CAD build for the part. Positions are in the model's coordinates, mm. A direction names the side the tool comes from. Round coordinates to 2 decimals unless told otherwise and drop trailing zeros. Write each loop counter-clockwise with the first axis right and the second up, starting at its lowest first coordinate (ties: lowest second). Pieces come first, ordered by that corner, then holes. Notation, with made-up numbers: (8, -34) - (14, -34) arc R7 ccw to (14, -22) - close; hole circle Ø9 at (13.5, -18.5). An arc over 180 degrees is marked (long way). Use one line per item in the form item = value. Start each with the question number.
Item 1: Drill centre lines: L1, parallel to Z at x = 15, y = 5.75; L2, parallel to Y at x = 27.5, z = -14.5. Where is each one in solid material? Low to high.
Item 2: Tool access for faces 4 (the cylindrical face through (9.4, 99.43, -24.65)), 5 (the cylindrical face through (15.18, 39.4, -34.43)), 6 (the cylindrical face through (12.05, 6.59, -20.2)), 7 (the cylindrical face through (0.57, 50.56, -10.29)): list every direction of +Z, -Z, +X, -X, +Y, -Y with a clear straight run to the whole face (end or side of a thin tool).
Item 3: Pull direction X, two halves, no side cores. Call faces 1 (the flat face through (15, 48, -50)), 2 (the cylindrical face through (0.6, 14.43, -17.28)), 3 (the flat face through (20, 86, -25)): +X half, -X half, draft (parallel to the pull), parting line (faces both ways), or undercut.
Item 4: Band-saw the part on B-B, the plane x = 4. List the corners of the cut face in (y, z).
Item 5: Pin check, flat tips, straight feed: pin 1 (13.5 mm diameter, centred on x = 17, z = -27.5, fed in from -Y); pin 2 (10.5 mm diameter, centred on x = 11.5, y = 30.5, fed in from +Z); pin 3 (6.5 mm diameter, centred on x = 15, z = -17.5, fed in from +Y). Stop position of each tip, or through.
Item 6: Band-saw the part on D-D, the plane z = -15. Give the number of separate pieces and of enclosed holes in the cut face, and give its area (3 significant figures).
Item 7: Band-saw the part on A-A, the plane y = 90. List the corners of the cut face in (x, z).
Item 8: Band-saw the part on C-C, the plane x = 15. List the corners of the cut face in (y, z), and give its area (3 significant figures).
from build123d import *

# Parameters (mm, degrees)
BOSS_EXTRUDE1_DEPTH = 30
SKETCH3_R           = 4
CUT_EXTRUDE1_DEPTH  = 30
SKETCH4_W           = 10
SKETCH4_H           = 50
CUT_EXTRUDE2_DEPTH  = 51
SKETCH5_R           = 2.5
CUT_EXTRUDE3_DEPTH  = 30
FILLET1_R           = 2
CUT_EXTRUDE4_DEPTH  = 31
FILLET2_R           = 2


with BuildPart() as part:
    # Sketch2 → Boss-Extrude1 (new body)
    with BuildSketch(Plane(origin=(0, 0, 0), x_dir=(0, 0, -1), z_dir=(1, 0, 0))):
        Polygon((0, 40), (35, 40), (35, 15), (0, 15), (0, 0), (50, 0), (50, 100), (0, 100), align=None)
    extrude(amount=BOSS_EXTRUDE1_DEPTH)

    # Sketch3 → Cut-Extrude1 (cut)
    with BuildSketch(Plane(origin=(0, 15, 0), x_dir=(1, 0, 0), z_dir=(0, 1, 0))):
        with Locations((15, 17.5)):
            Circle(SKETCH3_R)
    extrude(amount=-CUT_EXTRUDE1_DEPTH, mode=Mode.SUBTRACT)

    # Sketch4 → Cut-Extrude2 (cut, through all)
    with BuildSketch(Plane.XY):
        with Locations((15, 100)):
            Rectangle(SKETCH4_W, SKETCH4_H)
    extrude(amount=-CUT_EXTRUDE2_DEPTH, mode=Mode.SUBTRACT)

    # Sketch5 → Cut-Extrude3 (cut)
    with BuildSketch(Plane.ZY):
        with Locations((-35, 90)):
            Circle(SKETCH5_R)
        with Locations((-15, 90)):
            Circle(SKETCH5_R)
    extrude(amount=-CUT_EXTRUDE3_DEPTH, mode=Mode.SUBTRACT)

    # Fillet1
    fillet1_edges = [part.edges().sort_by_distance(p)[0] for p in [
        (11, 15, -17.5),
    ]]
    fillet(fillet1_edges, radius=FILLET1_R)

    # Sketch6 → Cut-Extrude4 (cut, through all)
    with BuildSketch(Plane.ZY):
        Polygon((-20, 40), (0, 60), (0, 40), align=None)
    extrude(amount=-CUT_EXTRUDE4_DEPTH, mode=Mode.SUBTRACT)

    # Fillet2
    fillet2_edges = [part.edges().sort_by_distance(p)[0] for p in [
        (30, 50, -50),
        (0, 100, -25),
        (15, 40, -35),
        (15, 15, -35),
        (15, 15, 0),
        (25, 100, -50),
        (25, 100, 0),
        (30, 7.5, 0),
        (30, 15, -17.5),
        (30, 27.5, -35),
        (5, 100, 0),
        (5, 100, -50),
        (10, 100, -25),
        (20, 100, -25),
        (30, 100, -25),
        (0, 80, 0),
        (0, 40, -27.5),
        (30, 80, 0),
        (30, 40, -27.5),
        (30, 50, -10),
        (15, 40, -20),
        (15, 60, 0),
        (0, 50, -10),
        (0, 27.5, -35),
        (0, 15, -17.5),
        (0, 7.5, 0),
        (0, 50, -50),
    ]]
    fillet(fillet2_edges, radius=FILLET2_R)


solid = part.part
Determined:
q1.L1 = -50 to -21.5, -13.5 to 0
q1.L2 = 0 to 15, 45.5 to 87.55, 92.45 to 100
q2.face_4 = +Z, -Z, +Y
q2.face_5 = +Z, +X, -X
q2.face_6 = -Y
q2.face_7 = +Z, -X
q3.face_1 = draft
q3.face_2 = -X half
q3.face_3 = undercut
q4.outline = (0, -50) - (98, -50) arc R2 ccw to (100, -48) - (100, -2) arc R2 ccw to (98, 0) - (60.83, 0) arc R2 ccw to (59.41, -0.59) - (40.59, -19.41) arc R2 ccw to (40, -20.83) - (40, -33) arc R2 cw to (38, -35) - (17, -35) arc R2 cw to (15, -33) - (15, -2) arc R2 ccw to (13, 0) - (0, 0) - close; hole circle Ø5 at (90, -35); hole circle Ø5 at (90, -15)
q5.pin_1 = 0
q5.pin_2 = -35
q5.pin_3 = 75
q6.separate_pieces = 5
q6.enclosed_holes = 0
q6.area = 1,650 mm²
q7.outline = (0, -48) arc R2 ccw to (2, -50) - (10, -50) - (10, -37.5) - (0, -37.5) - close; (0, -32.5) - (10, -32.5) - (10, -17.5) - (0, -17.5) - close; (0, -12.5) - (10, -12.5) - (10, 0) - (2, 0) arc R2 ccw to (0, -2) - close; (20, -50) - (28, -50) arc R2 ccw to (30, -48) - (30, -37.5) - (20, -37.5) - close; (20, -32.5) - (30, -32.5) - (30, -17.5) - (20, -17.5) - close; (20, -12.5) - (30, -12.5) - (30, -2) arc R2 ccw to (28, 0) - (20, 0) - close
q8.outline = (0, -50) - (75, -50) - (75, 0) - (60.83, 0) arc R2 ccw to (59.41, -0.59) - (40.59, -19.41) arc R2 ccw to (40, -20.83) - (40, -33) arc R2 cw to (38, -35) - (17, -35) arc R2 cw to (15, -33) - (15, -23.5) arc R2 ccw to (13, -21.5) - (0, -21.5) - close; (0, -13.5) - (13, -13.5) arc R2 ccw to (15, -11.5) - (15, -2) arc R2 ccw to (13, 0) - (0, 0) - close
q8.area = 2,550 mm²
